Read the model definition and answer for the solid it produces. Units are mm, in the model's axes. A direction names the side the tool comes from. Coordinates: 2 decimals unless noted, no trailing zeros. Order: outer loops, then holes, each group sorted by start corner. A loop starts at its lowest first (then second) coordinate and runs counter-clockwise, first axis right, second up. Notation, with made-up numbers: M -27.5,36.25 L 18.5,36.25 A19 ccw 18.5,71.25 Z; hole C 9.25,48.25 d7. An arc over 180 degrees is marked long. Put each result on its own line as item: value.
from build123d import *

# Parameters (mm, degrees)
SKETCH3_W           = 22.864276312
SKETCH3_H           = 28.163711354
CUT_EXTRUDE1_DEPTH  = 24.243278598
BOSS_EXTRUDE1_DEPTH = 1
SKETCH6_W           = 10.001476891
SKETCH6_H           = 0.625
BOSS_EXTRUDE2_DEPTH = 3.6
SKETCH7_W           = 10.001476891
SKETCH7_H           = 1.25
BOSS_EXTRUDE3_DEPTH = 0.5
BOSS_EXTRUDE4_DEPTH = 0.6
SKETCH9_W           = 10.001476891
SKETCH9_H           = 0.1
CUT_EXTRUDE2_DEPTH  = 4
CUT_EXTRUDE3_DEPTH  = 0.2
SKETCH12_W          = 10.001476891
SKETCH12_H          = 0.8
BOSS_EXTRUDE5_DEPTH = 0.6


with BuildPart() as part:
    # Sweep1: sweep along a path in Sketch2
    with BuildLine(Plane.XY) as sweep1_path:
        Line((0, 0), (-15, 15))
    # Sketch1 → Sweep1 (sweep)
    with BuildSketch(Plane(origin=(0, 0, 0), x_dir=(1, 0, 0), z_dir=(0, 1, 0))):
        with BuildLine():
            Line((0, 0), (9.3, 0))
            ThreePointArc((9.3, 0), (13.425, 4.125), (9.3, 8.25))
            Line((9.3, 8.25), (0, 8.25))
            Line((0, 8.25), (0, 9.5))
            Line((0, 9.5), (9.3, 9.5))
            ThreePointArc((9.3, 9.5), (14.675, 4.125), (9.3, -1.25))
            Line((9.3, -1.25), (0, -1.25))
            Line((0, -1.25), (0, 0))
        make_face()
    sweep(path=sweep1_path.line)

    # Sketch3 → Cut-Extrude1 (cut, through all)
    with BuildSketch(Plane(origin=(0, 0, 0), x_dir=(0, 0, -1), z_dir=(-1, 0, 0))):
        with Locations((2.794700938, -13.471268798)):
            Rectangle(SKETCH3_W, SKETCH3_H)
    extrude(amount=CUT_EXTRUDE1_DEPTH, mode=Mode.SUBTRACT)

    # Sketch5 → Boss-Extrude1 (add)
    with BuildSketch(Plane(origin=(0, 0, 0), x_dir=(0, 0, -1), z_dir=(-1, 0, 0))):
        with BuildLine():
            Line((9.5, 0), (9.5, -12.5))
            ThreePointArc((9.5, -12.5), (4.125, -17.875), (-1.25, -12.5))
            Line((-1.25, -12.5), (-1.25, 0))
            Line((-1.25, 0), (0, 0))
            Line((0, 0), (0, -9.3))
            ThreePointArc((0, -9.3), (4.125, -13.425), (8.25, -9.3))
            Line((8.25, -9.3), (8.25, 0))
            Line((8.25, 0), (9.5, 0))
        make_face()
    extrude(amount=BOSS_EXTRUDE1_DEPTH)

    # Sketch6 → Boss-Extrude2 (add)
    with BuildSketch(Plane.XZ):
        with Locations((4.000738446, -8.5625)):
            Rectangle(SKETCH6_W, SKETCH6_H)
        with Locations((4.000738446, 0.3125)):
            Rectangle(SKETCH6_W, SKETCH6_H)
    extrude(amount=BOSS_EXTRUDE2_DEPTH)

    # Sketch7 → Boss-Extrude3 (add)
    with BuildSketch(Plane.XZ.offset(3.6)):
        with Locations((4.000738446, 0.625)):
            Rectangle(SKETCH7_W, SKETCH7_H)
        with Locations((4.000738446, -8.875)):
            Rectangle(SKETCH7_W, SKETCH7_H)
    extrude(amount=BOSS_EXTRUDE3_DEPTH)

    # Sketch8 → Boss-Extrude4 (add)
    with BuildSketch(Plane(origin=(0, -1, 0), x_dir=(-1, 0, 0), z_dir=(0, -1, 0))):
        Polygon((-9.001476891, 8.25), (-9.001476891, 0), (-3.501476891, 0), (1, 0), (1, 0.8), (-3.501476891, 0.8), (-3.501476891, 2.875), (1, 2.875), (1, 5.375), (-3.501476891, 5.375), (-3.501476891, 7.45), (1, 7.45), (1, 8.25), (-3.501476891, 8.25), align=None)
    extrude(amount=BOSS_EXTRUDE4_DEPTH)

    # Sketch9 → Cut-Extrude2 (cut)
    with BuildSketch(Plane(origin=(0, 0.2, 0), x_dir=(-1, 0, 0), z_dir=(0, -1, 0))):
        with Locations((-4.000738446, -0.675)):
            Rectangle(SKETCH9_W, SKETCH9_H)
        with Locations((-4.000738446, 8.925)):
            Rectangle(SKETCH9_W, SKETCH9_H)
    extrude(amount=CUT_EXTRUDE2_DEPTH, mode=Mode.SUBTRACT)

    # Sketch10 → Cut-Extrude3 (cut)
    with BuildSketch(Plane.XZ):
        Polygon((9.001476891, 0.725), (9.001476891, -8.875), (9.001476891, -10.300951844), (15.96659325, -10.300951844), (15.96659325, 1.743519047), (9.001476891, 1.743519047), align=None)
    extrude(amount=-CUT_EXTRUDE3_DEPTH, mode=Mode.SUBTRACT)

    # Sketch12 → Boss-Extrude5 (add)
    with BuildSketch(Plane.XZ.offset(4.1)):
        with Locations((4.000738446, -7.85)):
            Rectangle(SKETCH12_W, SKETCH12_H)
        with Locations((4.000738446, -0.4)):
            Rectangle(SKETCH12_W, SKETCH12_H)
    extrude(amount=-BOSS_EXTRUDE5_DEPTH)


solid = part.part
Q1. Given pin 1 (6 mm diameter, centred on y = 5, z = -1, fed in from +X); pin 2 (2 mm diameter, centred on x = 10, z = -5, fed in from +Y); pin 3 (0.5 mm diameter, centred on x = 1, y = -1, fed in from -Z) (3 decimals), each flat-ended and moving along its own axis, determine where each tip first touches the part or whether it passes through.
Answers below:
pin 1: stops at x = 12.07
pin 2: stops at y = 5.61
pin 3: stops at z = -8.875
Q2. Find section A-A on y = -0.5. Write down the section's boundary in (x, z) (3 decimals), plus the area to 3 significant figures.
Answers below:
outline: M -1,-8.875 L 9.001,-8.875 L 9.001,-8.25 L -1,-8.25 Z; M -1,0 L 9.001,0 L 9.001,0.625 L -1,0.625 Z
area: 12.5 mm^2
Q3. A tool of negligible diameter and unlimited length cuts with its end or side. For faces 5 (the face through (13, 0.2, -7)), 6 (the face through (-0.493, 13.424, -4.034)), 7 (the face through (4, -3, -8.25)), from which of +Z, -Z, +X, -X, +Y, -Y can it reach the whole face along a straight path? Write none if from no direction.
Answers below:
face 5: +X
face 6: -X
face 7: +X, -X
Q4. For a pull along Z with two mould halves and no side action, classify faces 1 (the face through (4, -3.5, -8)), 2 (the face through (2, 4, 1.25)), 3 (the face through (2, 3, -9.5)), 4 (the face through (4, -4.1, 0)) as +Z half, -Z half, draft (parallel to the pull), parting line (faces both ways), or undercut.
Answers below:
face 1: undercut
face 2: +Z half
face 3: -Z half
face 4: draft
Q5. Consider line 1 along Z through (x, y) = (3, -1.5) (3 decimals); line 2 along Z through (x, y) = (7.75, -0.25) (3 decimals); line 3 along Y through (x, z) = (3, -7.5). Determine where each line is inside the solid, lowest interval first.
Answers below:
line 1: z = -8.875 to -7.45, -5.375 to -2.875, -0.8 to 0.625
line 2: z = -8.875 to -8.25, 0 to 0.625
line 3: y = -4.1 to -3.5, -1.6 to -1, 8.67 to 10.48
Q6. Find section B-B on y = 16.25. Write down the section's boundary in (x, z).
Answers below:
outline: M -1,-7.98 L 0,-7.98 L 0,-0.27 L -1,-0.27 Z
